Could you check a few things on this model? Use its own coordinates, in mm. Face numbers are marked on the shaded views. A direction names the side the tool comes from. Give positions to 0.01 mm unless a question says otherwise; leave off trailing zeros. Loops run counter-clockwise (first coordinate to the right, second up) from the corner with the lowest first, then second, coordinate; pieces in that order, holes last. Notation, with made-up numbers: (-30, 70.5) - (29, 70.5) arc R33 ccw to (29, 106.5) - close; hole circle Ø3 at (-22.75, 41.25). An arc over 180 degrees is marked (long way). Write each question's results on one line, items separated by ' | '. Start each with the question number.
1) I want a section at C-C, the plane y = 12.5. Write out the boundary of the cut face in (x, z).
2) If I drill on probe 1 along Y at (x, z) = (3.25, 0.25); probe 2 along Z at (x, y) = (1.5, 7); probe 3 along Z at (x, y) = (1, 14), over which ranges is the centre line in solid material (lowest first)? Write a range as [from, to].
3) If we mould it in two halves opening along X, with no side actions, what happens to the marked faces 3, 4, 5 and 6? For each: +X half, -X half, draft (parallel to the pull), parting line (faces both ways), or undercut.
4) I'm going to push flat-ended pins straight in: pin 1 (1 mm diameter, centred on x = 2.5, y = 5.5, fed in from -Z); pin 2 (1 mm diameter, centred on x = 1.5, y = 23.5, fed in from -Z); pin 3 (5 mm diameter, centred on y = 16.5, z = 3, fed in from -X). Where does each tip first touch, or does it pass through?
5) On a 3-axis mill with a long thin cutter (end or side, diameter ignored), from which of +Z, -Z, +X, -X, +Y, -Y can I reach the whole of each face in a straight line? I mean the marked faces 1 and 2. Say none if no direction works.
6) I want a section at A-A, the plane x = 0. Write out the boundary of the cut face in (y, z), and give its area (3 significant figures).
7) I want a section at B-B, the plane z = 0. Write out the boundary of the cut face in (x, y).
from build123d import *

# Parameters (mm, degrees)
SKETCH2_R           = 4.5
BOSS_EXTRUDE1_DEPTH = 1.5
SKETCH3_R           = 2.5
BOSS_EXTRUDE2_DEPTH = 30
CHAMFER1_SIZE       = 0.1
CHAMFER2_SIZE       = 0.75
CHAMFER2_SIZE2      = 0.3
CUT_EXTRUDE1_DEPTH  = 3
CHAMFER3_SIZE       = 0.3


with BuildPart() as part:
    # Sketch2 → Boss-Extrude1 (new body)
    with BuildSketch(Plane(origin=(0, 0, 0), x_dir=(1, 0, 0), z_dir=(0, 1, 0))):
        Circle(SKETCH2_R)
    extrude(amount=BOSS_EXTRUDE1_DEPTH)

    # Sketch3 → Boss-Extrude2 (add)
    with BuildSketch(Plane(origin=(0, 1.5, 0), x_dir=(1, 0, 0), z_dir=(0, 1, 0))):
        Circle(SKETCH3_R)
    extrude(amount=BOSS_EXTRUDE2_DEPTH)

    # Chamfer1
    chamfer1_edges = [part.edges().sort_by_distance(p)[0] for p in [
        (-2.5, 1.5, 0),
    ]]
    chamfer(chamfer1_edges, length=CHAMFER1_SIZE)

    # Chamfer2
    chamfer2_edges = [part.edges().sort_by_distance(p)[0] for p in [
        (-4.5, 0, 0),
    ]]
    chamfer2_side = [part.faces().sort_by_distance(p)[0] for p in [
        (0, 0, 0),
    ]]
    chamfer(chamfer2_edges, length=CHAMFER2_SIZE, length2=CHAMFER2_SIZE2, reference=chamfer2_side[0])

    # Sketch4 → Cut-Extrude1 (cut)
    with BuildSketch(Plane.XZ):
        Polygon((-0.422737578, 1.679670486), (-1.6660061, 0.473733761), (-1.243268521, -1.205936725), (0.422737578, -1.679670486), (1.6660061, -0.473733761), (1.243268521, 1.205936725), align=None)
    extrude(amount=-CUT_EXTRUDE1_DEPTH, mode=Mode.SUBTRACT)

    # Chamfer3
    chamfer3_edges = [part.edges().sort_by_distance(p)[0] for p in [
        (-2.5, 31.5, 0),
    ]]
    chamfer(chamfer3_edges, length=CHAMFER3_SIZE)


solid = part.part
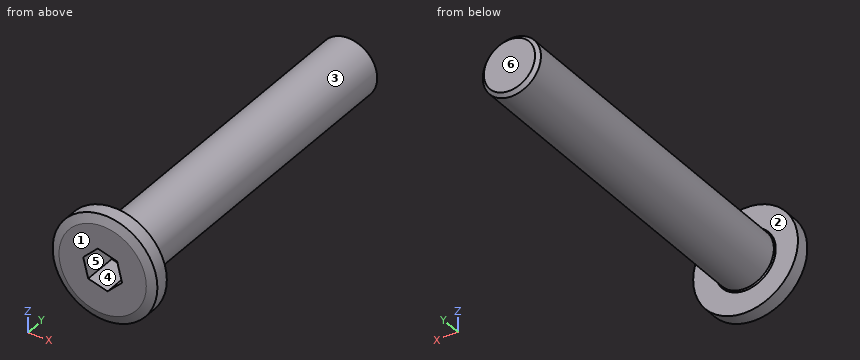
Answers:
1) outline: circle Ø5 at (0, 0)
2) probe 1: y = [0, 1.5] | probe 2: z = [-2, 2] | probe 3: z = [-2.29, 2.29]
3) face 3: parting line | face 4: undercut | face 5: undercut | face 6: draft
4) pin 1: stops at z = -1.5 | pin 2: stops at z = -2.29 | pin 3: stops at x = -2.45
5) face 1: +Z, -Z, +X, -X, -Y | face 2: +Y
6) outline: (0, -3.75) - (0.3, -4.5) - (1.5, -4.5) - (1.5, -2.6) - (1.6, -2.5) - (31.2, -2.5) - (31.5, -2.2) - (31.5, 2.2) - (31.2, 2.5) - (1.6, 2.5) - (1.5, 2.6) - (1.5, 4.5) - (0.3, 4.5) - (0, 3.75) - (0, 1.56) - (3, 1.56) - (3, -1.56) - (0, -1.56) - close | area: 154 mm2
7) outline: (-4.5, 0.3) - (-3.75, 0) - (-1.55, 0) - (-1.55, 3) - (1.55, 3) - (1.55, 0) - (3.75, 0) - (4.5, 0.3) - (4.5, 1.5) - (2.6, 1.5) - (2.5, 1.6) - (2.5, 31.2) - (2.2, 31.5) - (-2.2, 31.5) - (-2.5, 31.2) - (-2.5, 1.6) - (-2.6, 1.5) - (-4.5, 1.5) - close
